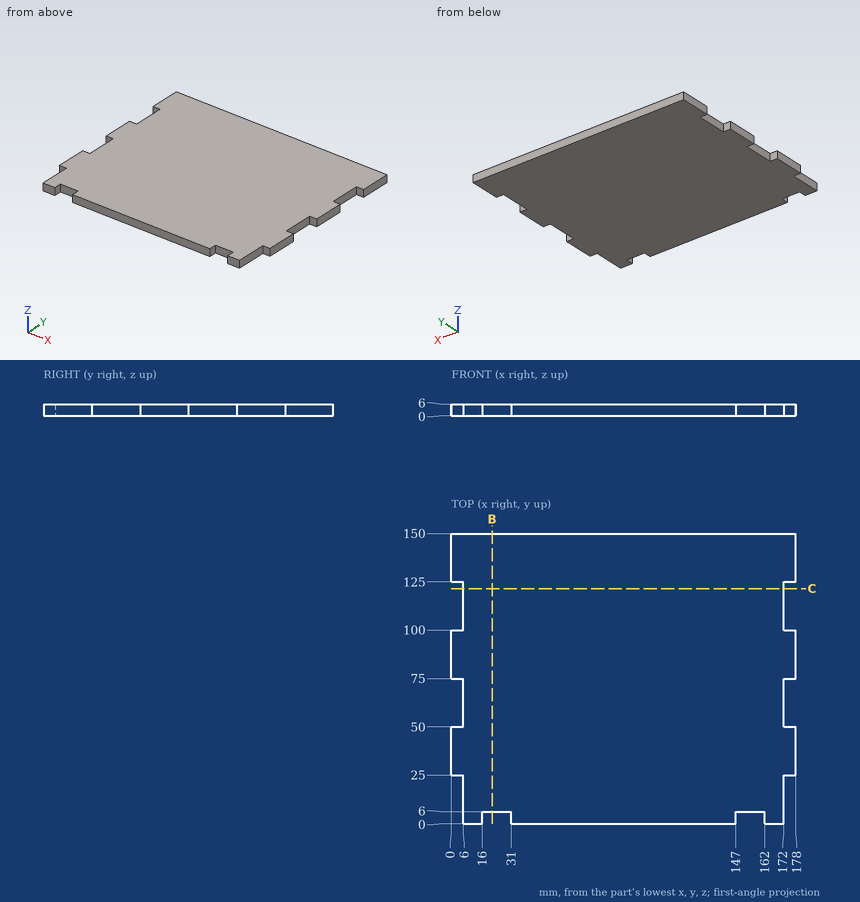
Study the drawing (mm; zero at the part's minimum x, y, z) and answer. Give positions to 0.01 mm unless a question says otherwise; leave off trailing zeros. Order: outer loops, then holes, each group sorted by start corner. A loop starts at its lowest first (then second) coordinate and runs counter-clockwise, first axis right, second up.
1) Consider line 1 along X through (y, z) = (57, 1.75); line 2 along Y through (x, z) = (152, 1). Determine where each line is inside the solid, lowest interval first.
Reported:
line 1: x = 6 to 172
line 2: y = 6 to 150
2) Given P1, Ø1.8, axis at x = 2, z = 3, coming from the -Y side; P2, Ø1.8, axis at x = 25, z = 4, coming from the -Y side; P3, Ø1.8, axis at y = 10.5, z = 3, coming from the +X side, each flat-ended and moving along its own axis, determine where each tip first touches the part or whether it passes through.
Reported:
P1: stops at y = 25
P2: stops at y = 6
P3: stops at x = 172
3) Find section C-C on y = 121.5. Write down the section's boundary in (x, z), then the cut area to 3 significant figures.
Reported:
outline: (6, 0) - (172, 0) - (172, 6) - (6, 6) - close
area: 996 mm2
4) Find section B-B on x = 21. Write down the section's boundary in (y, z), then the cut area to 3 significant figures.
Reported:
outline: (6, 0) - (150, 0) - (150, 6) - (6, 6) - close
area: 864 mm2
